```python
from build123d import *

# Parameters (mm, degrees)
SKETCH_1_W             = 35.5
SKETCH_1_H             = 33.5
EXTRUDE_227_DEPTH      = 2.5
SKETCH_3_W             = 14.5
SKETCH_3_H             = 3
EXTRUDE_815_DEPTH      = 1.5
SKETCH_4_W             = 14.5
SKETCH_4_H             = 1
CUT_EXTRUDE_1043_DEPTH = 25.533140851
SKETCH_5_R             = 1.4
CUT_EXTRUDE_2_DEPTH    = 25.533140851
SKETCH_6_R             = 1.4
CUT_EXTRUDE_3_DEPTH    = 25.533140851


with BuildPart() as part:
    # 草图1 → Extrude 227 (new body)
    with BuildSketch(Plane.XY):
        Rectangle(SKETCH_1_W, SKETCH_1_H)
    extrude(amount=EXTRUDE_227_DEPTH)

    # 草图3 → Extrude 815 (add)
    with BuildSketch(Plane.XY.offset(2.5)):
        Polygon((-17.75, 10.75), (-17.75, -12.75), (-7.25, -12.75), (7.25, -12.75), (17.75, -12.75), (17.75, 10.75), align=None)
        with Locations((0, -14.25)):
            Rectangle(SKETCH_3_W, SKETCH_3_H)
    extrude(amount=EXTRUDE_815_DEPTH)

    # 草图4 → Cut-Extrude 1043 (cut, through all)
    with BuildSketch(Plane.XY.offset(2.5)):
        with Locations((0, -16.25)):
            Rectangle(SKETCH_4_W, SKETCH_4_H)
    extrude(amount=-CUT_EXTRUDE_1043_DEPTH, mode=Mode.SUBTRACT)

    # 草图5 → 切除-拉伸2 (cut, through all)
    with BuildSketch(Plane.XY.offset(2.5)):
        with Locations((15.35, 13.65)):
            Circle(SKETCH_5_R)
        with Locations(Location((-15.35, 13.65, 0), (0, 0, 180))):
            Circle(SKETCH_5_R)
    extrude(amount=-CUT_EXTRUDE_2_DEPTH, mode=Mode.SUBTRACT)

    # 草图6 → 切除-拉伸3 (cut, through all)
    with BuildSketch(Plane.XY.offset(2.5)):
        with Locations((15.35, -14.95)):
            Circle(SKETCH_6_R)
    cut_extrude_3 = extrude(amount=-CUT_EXTRUDE_3_DEPTH, mode=Mode.SUBTRACT)

    # 镜向1: 切除-拉伸3 across plane
    add(cut_extrude_3.mirror(Plane(origin=(0, 0, 0), x_dir=(0, 0, 1), z_dir=(1, 0, 0))), mode=Mode.SUBTRACT)


solid = part.part
```
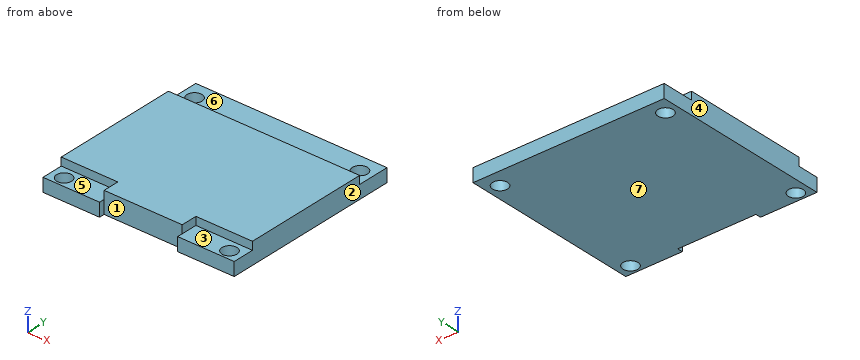
Input: part model. Units: mm. Frame: model coordinates. Face numbers are marked on the shaded views. A direction names the side the tool comes from. Give positions to 0.01 mm unless a question says otherwise; leave off trailing zeros. Loops run counter-clockwise (first coordinate to the right, second up) from the corner with the lowest first, then second, coordinate; pieces in that order, holes last.
1) Contact query for flat-ended pins moving along their axis: pin 1 (0.8 mm diameter, centred on x = -11, z = 3.5, fed in from -Y); pin 2 (0.8 mm diameter, centred on y = -14.5, z = 3.5, fed in from -X); pin 3 (5 mm diameter, centred on x = -1, y = 15, fed in from +Z). Output: stop coordinate, or through.
A:
pin 1: stops at y = -12.75
pin 2: stops at x = -7.25
pin 3: stops at z = 2.5
2) Line query: L1, parallel to Y at x = -15.35, z = 1; L2, parallel to Z at x = 11, y = 15; L3, parallel to Y at x = 2, z = 1.7. Output: solid intervals per line, ascending.
A:
L1: y = -16.75 to -16.35, -13.55 to 12.25, 15.05 to 16.75
L2: z = 0 to 2.5
L3: y = -15.75 to 16.75
3) Section query B-B on x = -15.35. Return the cut outline in (y, z), and give its area (3 significant figures).
A:
outline: (-16.75, 0) - (-16.35, 0) - (-16.35, 2.5) - (-16.75, 2.5) - close; (-13.55, 0) - (12.25, 0) - (12.25, 2.5) - (10.75, 2.5) - (10.75, 4) - (-12.75, 4) - (-12.75, 2.5) - (-13.55, 2.5) - close; (15.05, 0) - (16.75, 0) - (16.75, 2.5) - (15.05, 2.5) - close
area: 105 mm2
4) Section query C-C on z = 1.95. Return the cut outline in (x, y).
A:
outline: (-17.75, -16.75) - (-7.25, -16.75) - (-7.25, -15.75) - (7.25, -15.75) - (7.25, -16.75) - (17.75, -16.75) - (17.75, 16.75) - (-17.75, 16.75) - close; hole circle Ø2.8 at (-15.35, -14.95); hole circle Ø2.8 at (-15.35, 13.65); hole circle Ø2.8 at (15.35, -14.95); hole circle Ø2.8 at (15.35, 13.65)
5) Section query A-A on y = 13.65. Return the cut outline in (x, z), and give its area (4 significant figures).
A:
outline: (-17.75, 0) - (-16.75, 0) - (-16.75, 2.5) - (-17.75, 2.5) - close; (-13.95, 0) - (13.95, 0) - (13.95, 2.5) - (-13.95, 2.5) - close; (16.75, 0) - (17.75, 0) - (17.75, 2.5) - (16.75, 2.5) - close
area: 74.75 mm2
6) Section query D-D on x = 9.5. Return the cut outline in (y, z), and give its area (3 significant figures).
A:
outline: (-16.75, 0) - (16.75, 0) - (16.75, 2.5) - (10.75, 2.5) - (10.75, 4) - (-12.75, 4) - (-12.75, 2.5) - (-16.75, 2.5) - close
area: 119 mm2
7) Reachability of the marked faces 5, 6 and 7 from +Z, -Z, +X, -X, +Y, -Y: full face, straight path, thin tool, end or side. Return the list, or none.
A:
face 5: +Z, -X, -Y
face 6: +Z, +X, -X, +Y
face 7: -Z, +X, -X, +Y, -Y
8) Mould query, pull axis X, two halves, no side actions, for the marked faces 1, 2, 3 and 4. Classes: released by +X, released by -X, zero draft, split by the parting line, or undercut.
A:
face 1: undercut
face 2: released by +X
face 3: zero draft
face 4: released by -X
